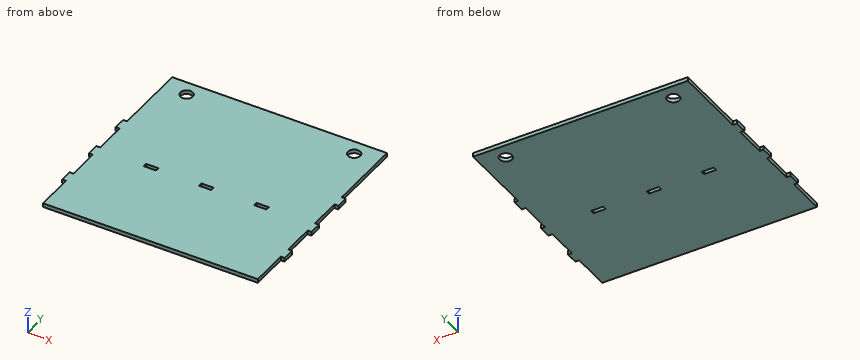
```python
from build123d import *

# Parameters (mm, degrees)
CROQUIS1_W              = 350
CROQUIS1_H              = 350
SALIENTE_EXTRUIR1_DEPTH = 6.35
CROQUIS2_W              = 6.35
CROQUIS2_H              = 20
SALIENTE_EXTRUIR2_DEPTH = 6.35
CROQUIS3_W              = 20
CROQUIS3_H              = 6.35
CORTAR_EXTRUIR1_DEPTH   = 10
CROQUIS4_R              = 10
CORTAR_EXTRUIR2_DEPTH   = 253.097491062


with BuildPart() as part:
    # Croquis1 → Saliente-Extruir1 (new body)
    with BuildSketch(Plane.XY):
        Rectangle(CROQUIS1_W, CROQUIS1_H)
    extrude(amount=SALIENTE_EXTRUIR1_DEPTH)

    # Croquis2 → Saliente-Extruir2 (add)
    with BuildSketch(Plane.ZY.offset(175)):
        with Locations((3.175, 42.5)):
            Rectangle(CROQUIS2_W, CROQUIS2_H)
        with Locations((3.175, -30)):
            Rectangle(CROQUIS2_W, CROQUIS2_H)
        with Locations((3.175, -102.5)):
            Rectangle(CROQUIS2_W, CROQUIS2_H)
    saliente_extruir2 = extrude(amount=SALIENTE_EXTRUIR2_DEPTH)

    # Simetría1: Saliente-Extruir2 across plane
    add(saliente_extruir2.mirror(Plane(origin=(0, 0, 0), x_dir=(0, 0, 1), z_dir=(1, 0, 0))))

    # Croquis3 → Cortar-Extruir1 (cut)
    with BuildSketch(Plane.XY.offset(6.35)):
        with Locations((0, -23.665)):
            Rectangle(CROQUIS3_W, CROQUIS3_H)
        with Locations((90, -23.665)):
            Rectangle(CROQUIS3_W, CROQUIS3_H)
        with Locations((-90, -23.665)):
            Rectangle(CROQUIS3_W, CROQUIS3_H)
    extrude(amount=-CORTAR_EXTRUIR1_DEPTH, mode=Mode.SUBTRACT)

    # Croquis4 → Cortar-Extruir2 (cut, through all)
    with BuildSketch(Plane.XY.offset(6.35)):
        with Locations((-136.525, 150)):
            Circle(CROQUIS4_R)
        with Locations((136.525, 150)):
            Circle(CROQUIS4_R)
    extrude(amount=-CORTAR_EXTRUIR2_DEPTH, mode=Mode.SUBTRACT)


solid = part.part
```
Work out the finished part from the listing and answer in its coordinate system (mm). Give positions to 0.01 mm unless a question says otherwise; leave off trailing zeros. Write each loop counter-clockwise with the first axis right and the second up, starting at its lowest first coordinate (ties: lowest second). Pieces come first, ordered by that corner, then holes. Notation, with made-up numbers: (38.5, -40) - (58.5, -40) arc R21 ccw to (58.5, -11) - close; hole circle Ø11 at (76, 12). An arc over 180 degrees is marked (long way). Use one line per item in the form item = value.
1. A cutting plane is placed at C-C (z = 1). State how many separate pieces and enclosed holes the cut face has, and give its area (3 significant figures).
Filled in:
separate_pieces = 1
enclosed_holes = 5
area = 122,000 mm^2
2. A cutting plane is placed at B-B (y = -148). Write down the section's boundary in (x, z), and give its area (3 significant figures).
Filled in:
outline = (-175, 0) - (175, 0) - (175, 6.35) - (-175, 6.35) - close
area = 2,220 mm^2
3. Consider L1, parallel to X at y = 151, z = 5; L2, parallel to Y at x = -97, z = 3; L3, parallel to X at y = -132.5, z = 1.25. Determine where each line is inside the solid, lowest interval first.
Filled in:
L1 = -175 to -146.47, -126.58 to 126.58, 146.47 to 175
L2 = -175 to -26.84, -20.49 to 175
L3 = -175 to 175
4. Each of these flat-tipped pins is pushed along its axis until it touches: pin 1 Ø3 at (y, z) = (1, 3) entering from -X; pin 2 Ø3 at (y, z) = (119.5, 3) entering from +X; pin 3 Ø3 at (x, z) = (-177, 2.5) entering from -Y. Where does it stop, or does it pass through?
Filled in:
pin_1 = -175
pin_2 = 175
pin_3 = -112.5
5. A cutting plane is placed at A-A (y = 150). Write down the section's boundary in (x, z) (3 decimals).
Filled in:
outline = (-175, 0) - (-146.525, 0) - (-146.525, 6.35) - (-175, 6.35) - close; (-126.525, 0) - (126.525, 0) - (126.525, 6.35) - (-126.525, 6.35) - close; (146.525, 0) - (175, 0) - (175, 6.35) - (146.525, 6.35) - close
